Geometry: final body of the model. Coordinates: model frame, mm. Give positions to 0.01 mm unless a question says otherwise; leave off trailing zeros. Order: outer loops, then holes, each group sorted by start corner. A loop starts at its lowest first (then second) coordinate and runs counter-clockwise, first axis right, second up. Notation, with made-up numbers: (51, -17.75) - (75, -17.75) arc R23 ccw to (75, 1.25) - close; hole circle Ø7 at (66.5, 81.5). An arc over 180 degrees is marked (long way). Put each result on its own line as item: value. Start each with the question number.
1. Section B-B on z = 10. Return the cut outline in (x, y).
2. First-contact query: P1, Ø1.9, axis at y = 0, z = 57, coming from the -X side; P2, Ø3.5, axis at x = -0.5, z = 28.5, coming from the +Y side; P3, Ø3.5, axis at x = 0.5, z = 38, coming from the -Y side. Flat tips, straight axial feed; report the tip coordinate or a pass-through.
3. Ray query, line 1 along X through (y, z) = (-0.25, 33); line 2 along X through (y, z) = (0.9, 127.5); line 3 along X through (y, z) = (0.8, 145). Return the intervals inside material, ascending. Write a range as from..to.
4. Section C-C on x = 11. Return the cut outline in (y, z).
5. Section A-A on y = 0.05. Return the cut outline in (x, z).
6. Mould query, pull axis Z, two halves, no side actions, for faces 1 (the cylindrical face through (35.096, -0.022, 101.57)), 2 (the flat face through (0, -1.191, 45)). Classes: pulls with the +Z half, pulls with the -Z half, needs draft (parallel to the pull), parting line crosses it, or undercut.
from build123d import *

# Parameters (mm, degrees)
F1_DEPTH = 1.5875
F2_DEPTH = 1.190625


with BuildPart() as f1:
    # F0 (on Front) → F1 (new body, symmetric)
    with BuildSketch(Plane.XZ):
        Polygon((-19.440318, 96.952444), (0, 88.9), (19.440318, 96.952444), (27.492762, 116.392762), (19.440318, 135.83308), (0, 143.885524), (-19.440318, 135.83308), (-27.492762, 116.392762), align=None)
        with BuildLine():
            Line((1.5875, 88.9), (1.5875, 85.124308))
            ThreePointArc((1.5875, 85.124308), (16.396635, 82.159273), (19.440318, 96.952444))
            Line((19.440318, 96.952444), (0, 88.9))
            Line((0, 88.9), (1.5875, 88.9))
        make_face()
        with BuildLine():
            Line((27.492762, 116.392762), (19.440318, 96.952444))
            ThreePointArc((19.440318, 96.952444), (35.19981, 101.812523), (27.492762, 116.392762))
        make_face()
        with BuildLine():
            Line((19.440318, 135.83308), (27.492762, 116.392762))
            ThreePointArc((27.492762, 116.392762), (35.19981, 130.973001), (19.440318, 135.83308))
        make_face()
        with BuildLine():
            Line((0, 143.885524), (19.440318, 135.83308))
            ThreePointArc((19.440318, 135.83308), (14.580239, 151.592572), (0, 143.885524))
        make_face()
        with BuildLine():
            ThreePointArc((0, 143.885524), (-14.580239, 151.592572), (-19.440318, 135.83308))
            Line((-19.440318, 135.83308), (0, 143.885524))
        make_face()
        with BuildLine():
            ThreePointArc((-19.440318, 135.83308), (-35.19981, 130.973001), (-27.492762, 116.392762))
            Line((-27.492762, 116.392762), (-19.440318, 135.83308))
        make_face()
        with BuildLine():
            ThreePointArc((-27.492762, 116.392762), (-35.19981, 101.812523), (-19.440318, 96.952444))
            Line((-19.440318, 96.952444), (-27.492762, 116.392762))
        make_face()
        with BuildLine():
            Line((-1.5875, 88.9), (0, 88.9))
            Line((0, 88.9), (-19.440318, 96.952444))
            ThreePointArc((-19.440318, 96.952444), (-16.396635, 82.159273), (-1.5875, 85.124308))
            Line((-1.5875, 85.124308), (-1.5875, 88.9))
        make_face()
        with BuildLine():
            ThreePointArc((0, 88.9), (0.61154, 86.935543), (1.5875, 85.124308))
            Line((1.5875, 85.124308), (1.5875, 88.9))
            Line((1.5875, 88.9), (0, 88.9))
        make_face()
        with BuildLine():
            ThreePointArc((-1.5875, 85.124308), (-0.61154, 86.935543), (0, 88.9))
            Line((0, 88.9), (-1.5875, 88.9))
            Line((-1.5875, 88.9), (-1.5875, 85.124308))
        make_face()
    extrude(amount=F1_DEPTH, both=True)

    # F0 (on Front) → F2 (join, symmetric)
    with BuildSketch(Plane.XZ):
        with BuildLine():
            Line((-1.5875, 0), (1.5875, 0))
            Line((1.5875, 0), (1.5875, 85.124308))
            ThreePointArc((1.5875, 85.124308), (0.61154, 86.935543), (0, 88.9))
            ThreePointArc((0, 88.9), (-0.61154, 86.935543), (-1.5875, 85.124308))
            Line((-1.5875, 85.124308), (-1.5875, 0))
        make_face()
    extrude(amount=F2_DEPTH, both=True)


solid = f1.part
Resolved:
1. outline: (-1.59, -1.19) - (1.59, -1.19) - (1.59, 1.19) - (-1.59, 1.19) - close
2. P1: x = -1.59
2. P2: y = 1.19
2. P3: y = -1.19
3. line 1: -1.59..1.59
3. line 2: -36..36
3. line 3: -20.67..-0.3, 0.3..20.67
4. outline: (-1.59, 80.39) - (1.59, 80.39) - (1.59, 152.4) - (-1.59, 152.4) - close
5. outline: (-27.49, 116.39) arc R10.71 ccw (long way) to (-19.44, 96.95) arc R10.71 ccw to (-1.59, 85.12) - (-1.59, 0) - (1.59, 0) - (1.59, 85.12) arc R10.71 ccw to (19.44, 96.95) arc R10.71 ccw (long way) to (27.49, 116.39) arc R10.71 ccw (long way) to (19.44, 135.83) arc R10.71 ccw (long way) to (0, 143.89) arc R10.71 ccw (long way) to (-19.44, 135.83) arc R10.71 ccw (long way) to start
6. face 1: undercut
6. face 2: needs draft
